Geometry: final body of the model. Coordinates: model frame, mm. Coordinates: 2 decimals unless noted, no trailing zeros. Order: outer loops, then holes, each group sorted by start corner. A loop starts at its lowest first (then second) coordinate and runs counter-clockwise, first axis right, second up. Notation, with made-up numbers: M 47,38 L 88,38 A11 ccw 88,53 Z; hole C 34.25,73 d3. An arc over 180 degrees is marked long. One line per question, with ' | ' between items.
Autodesk Inventor part; units mm, degrees
ref_plane "YZ Plane" through (0, 0, 0) normal (1, 0, 0) x (0, 1, 0)
ref_plane "XZ Plane" through (0, 0, 0) normal (0, 1, 0) x (-1, 0, 0)
ref_plane "XY Plane" through (0, 0, 0) normal (0, 0, 1) x (1, 0, 0)
sketch "Sketch1" plane through (0, 0, 0) normal (0, 0, 1) x (1, 0, 0)
  circle A0 centre (0, 0) radius 2.5
  dimension "d0" = 5
extrude "Extrusion1" add sketch "Sketch1" along normal blind 50
sketch "Sketch2" plane through (0, 0, 50) normal (0, 0, 1) x (1, 0, 0)
  circle A0 centre (0, 0) radius 1.1
  dimension "d3" = 2.2
extrude "Extrusion2" cut sketch "Sketch2" against normal blind 20
sketch "Sketch3" plane through (0, 0, 0) normal (0, 0, -1) x (-1, 0, 0)
  circle A0 centre (0, 0) radius 1.1
extrude "Extrusion3" cut sketch "Sketch3" against normal blind 20
thread "Thread1"
thread "Thread2"
properties part number "AxisLinear"
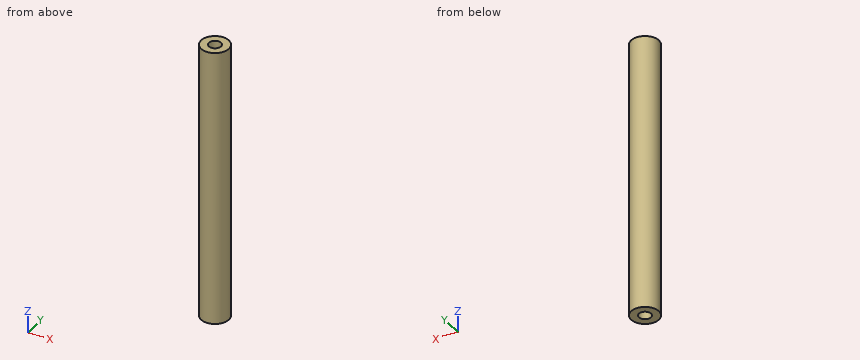
1. Section B-B, the plane z = 34. Output: boundary loops of the cut face in (x, y), and give its area (3 significant figures).
Response values:
outline: C 0,0 d5; hole C 0,0 d2.2 | area: 15.8 mm^2
2. Material intervals for line 1 (Y direction, x = 0, z = 35); line 2 (X direction, y = 0.4, z = 41.5), sorted ascending. Write a range as [from, to].
Response values:
line 1: y = [-2.5, -1.1], [1.1, 2.5] | line 2: x = [-2.47, -1.02], [1.02, 2.47]
3. Section A-A, the plane x = 0. Output: boundary loops of the cut face in (y, z), and give its area (3 significant figures).
Response values:
outline: M -2.5,0 L -1.1,0 L -1.1,20 L 1.1,20 L 1.1,0 L 2.5,0 L 2.5,50 L 1.1,50 L 1.1,30 L -1.1,30 L -1.1,50 L -2.5,50 Z | area: 162 mm^2
4. Pin query (flat end, axial travel): P1, Ø1.1, axis at x = -0.5, y = 0, coming from the +Z side; P2, Ø2, axis at x = 0, y = 0, coming from the -Z side; P3, Ø2, axis at y = 2, z = 20, coming from the -X side. Return the tip coordinate at first contact, or that it passes through.
Response values:
P1: stops at z = 30 | P2: stops at z = 20 | P3: stops at x = -2.29
5. Section D-D, the plane x = -1.9. Output: boundary loops of the cut face in (y, z).
Response values:
outline: M -1.62,0 L 1.62,0 L 1.62,50 L -1.62,50 Z
